For this review, use the dimensioned drawing (mm, ordinates from the lowest corner) and the shaded views. Round coordinates to 2 decimals unless told otherwise and drop trailing zeros. Loops run counter-clockwise (first coordinate to the right, second up) from the corner with the lowest first, then second, coordinate; pieces in that order, holes last. Notation, with made-up numbers: (77.5, 85) - (124.5, 85) arc R26 ccw to (124.5, 112) - close; hole circle Ø2 at (-26, 39.25). An arc over 180 degrees is marked (long way). Return JSON: item names as keys, results as strings. Group by question number.
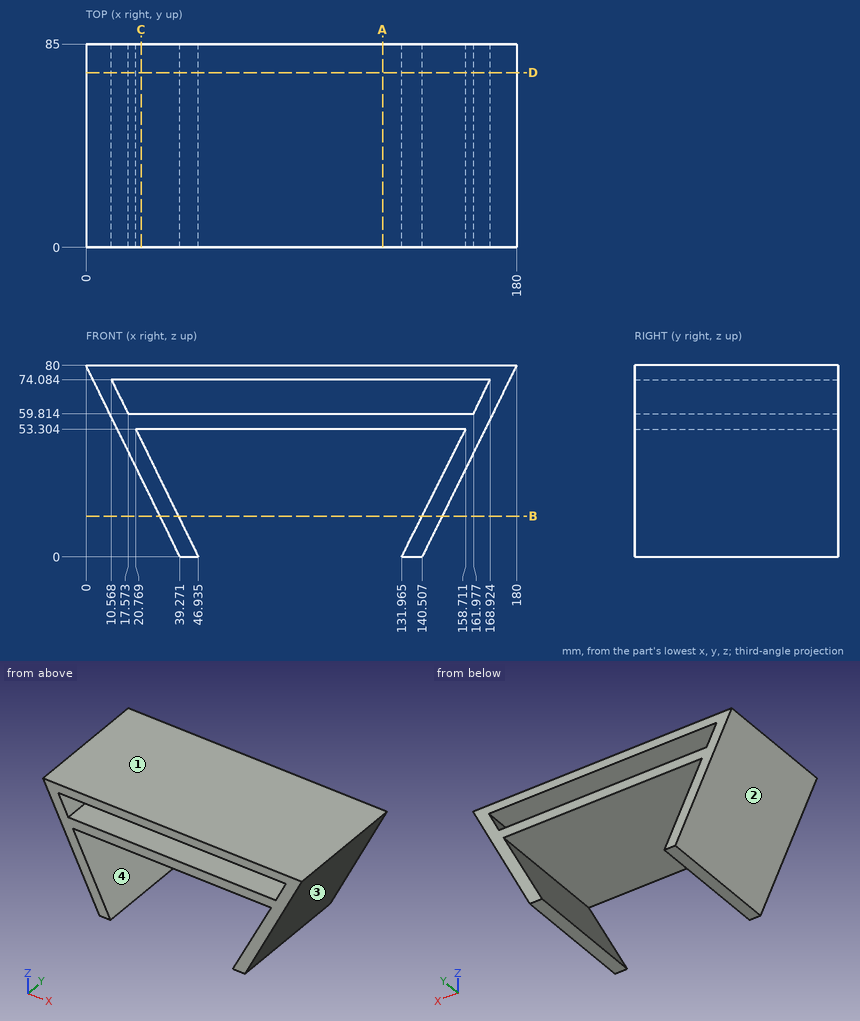
Q1. For line 1 (Z direction, x = 121.5, y = 6.5) (1 decimal); line 2 (Z direction, x = 31.5, y = 51) (1 decimal); line 3 (Z direction, x = 144, y = 44) (1 decimal), list the stretches that pass through material, from the lowest coordinate up.
Q2. Add section A-A, the plane x = 124. State the section outline as (y, z) points (1 decimal), plus the area to 3 significant figures.
Q3. Add section C-C, the plane x = 23. State the section outline as (y, z) points (1 decimal).
Q4. Draft analysis for pull direction X (two halves, no side actions). For the marked faces 1, 2, 3 and 4, state which applies: pulls with the +X half, pulls with the -X half, needs draft (parallel to the pull), parting line crosses it, or undercut.
Q5. Add section D-D, the plane y = 73. State the section outline as (x, z) points (1 decimal).
Q6. Add section B-B, the plane z = 17. State the section outline as (x, y) points (1 decimal), plus the area to 3 significant figures.
Q7. Insertion check: pin 1 Ø4 at (y, z) = (14.5, 49.5) entering from -X; pin 2 Ø4 at (y, z) = (12.5, 28) entering from +X; pin 3 Ø12 at (y, z) = (44.5, 46) entering from -X (1 decimal). Each pin has a flat end and moves straight along its axis. Give the tip position at first contact, or say it passes through.
Evaluation:
{
 "1": {"line 1": "53.3 to 59.8, 74.1 to 80", "line 2": "15.8 to 31.4, 53.3 to 59.8, 74.1 to 80", "line 3": "7.1 to 24, 53.3 to 59.8, 74.1 to 80"},
 "2": {"outline": "(0, 53.3) - (85, 53.3) - (85, 59.8) - (0, 59.8) - close; (0, 74.1) - (85, 74.1) - (85, 80) - (0, 80) - close", "area": "1,060 mm²"},
 "3": {"outline": "(0, 33.1) - (85, 33.1) - (85, 48.8) - (0, 48.8) - close; (0, 53.3) - (85, 53.3) - (85, 59.8) - (0, 59.8) - close; (0, 74.1) - (85, 74.1) - (85, 80) - (0, 80) - close"},
 "4": {"face 1": "needs draft", "face 2": "pulls with the -X half", "face 3": "pulls with the +X half", "face 4": "undercut"},
 "5": {"outline": "(0, 80) - (39.3, 0) - (46.9, 0) - (20.8, 53.3) - (158.7, 53.3) - (132, 0) - (140.5, 0) - (180, 80) - close; hole (10.6, 74.1) - (17.6, 59.8) - (162, 59.8) - (168.9, 74.1) - close"},
 "6": {"outline": "(30.9, 0) - (38.6, 0) - (38.6, 85) - (30.9, 85) - close; (140.5, 0) - (148.9, 0) - (148.9, 85) - (140.5, 85) - close", "area": "1,370 mm²"},
 "7": {"pin 1": "x = 13.99", "pin 2": "x = 155.32", "pin 3": "x = 13.7"}
}
